Autodesk Inventor part; units mm, degrees
ref_plane "Work Plane1" through (83, 0, 0) normal (-1, 0, 0) x (0, 0, 1)
ref_plane "YZ Plane" through (0, 0, 0) normal (1, 0, 0) x (0, 1, 0)
ref_plane "XZ Plane" through (0, 0, 0) normal (0, 1, 0) x (-1, 0, 0)
sketch "Sketch1" plane through (0, 0, 0) normal (0, 0, 1) x (1, 0, 0)
  line L0 (0, 0) -> (5, 0)
  line L1 (5, 0) -> (5, -18)
  line L2 (5, -18) -> (26, -18)
  line L3 (26, -18) -> (26, 0)
  line L4 (26, 0) -> (74, 0)
  arc A0 (74, 0) -> (74, 18) centre (74, 9) ccw
  line L5 (74, 18) -> (0, 18)
  line L6 (0, 18) -> (0, 0)
  circle A1 centre (20.5, -18) radius 10.5
  dimension "d0" = 5
  dimension "d1" = 18
  dimension "d2" = 21
  dimension "d3" = 18
  dimension "d4" = 48
  dimension "d5" = 18
  dimension "d6" = 9
  dimension "d7" = 74
  dimension "d8" = 21
extrude "Extrusion1" add sketch "Sketch1" along normal blind 6
sketch "Sketch2" plane through (0, 0, 0) normal (0, 0, -1) x (-1, 0, 0)
  circle A0 centre (-74, 9) radius 4.5
  arc A1 (-26, -9.0557) -> (-10, -18) centre (-20.5, -18) ccw
  circle A2 centre (-20.5, -18) radius 4.5
  point P0 (0, 0)
  dimension "d11" = 9
  dimension "d12" = 9
extrude "Extrusion2" cut sketch "Sketch2" against normal through all
sketch "Sketch3" plane through (0, 0, 0) normal (0, 0, -1) x (-1, 0, 0)
  circle A0 centre (-7, 9) radius 1.5
  circle A1 centre (-19, 9) radius 1.5
  point P0 (0, 0)
  dimension "d16" = 3
  dimension "d17" = 3
extrude "Extrusion3" cut sketch "Sketch3" against normal through all
ref_plane "Work Plane1" through (83, 0, 0) normal (-1, 0, 0) x (0, 0, 1)
sketch "Sketch4" plane through (83, 0, 0) normal (-1, 0, 0) x (0, 0, 1)
  circle A0 centre (3, 9) radius 1.5
  point P0 (0, 0)
  dimension "d22" = 3
extrude "Extrusion4" cut sketch "Sketch4" along normal blind 18
fillet "Fillet3" radius 1 8 edges at (83, 9, 0) (50, 0, 0) (37, 18, 0) (2.5, 0, 0) (5, -9, 0) (25.6235, -27.1652, 0) (7.5, -18, 0) (26, -4.5279, 0)
sketch "Sketch5" plane through (0, 18, 6) normal (0, 1, 0) x (1, 0, 0)
  circle A0 centre (69, 2.5) radius 1.5
  circle A1 centre (58, 2.5) radius 1.5
  point P0 (0, 6)
  dimension "d26" = 3
  dimension "d27" = 3
extrude "Extrusion5" cut sketch "Sketch5" against normal blind 5
sketch "Sketch6" plane through (0, 0, 6) normal (0, 0, 1) x (1, 0, 0)
  line L0 (71, 0) -> (77, 0)
  line L1 (77, 0) -> (77, 6)
  line L2 (77, 6) -> (71, 6)
  line L3 (71, 6) -> (71, 0)
  line L4 (17.5, -18) -> (23.5, -18)
  line L5 (23.5, -18) -> (23.5, -29)
  line L6 (23.5, -29) -> (17.5, -29)
  line L7 (17.5, -29) -> (17.5, -18)
  point P0 (0, 0)
  dimension "d30" = 6
  dimension "d31" = 6
  dimension "d32" = 6
  dimension "d33" = 11
extrude "Extrusion6" cut sketch "Sketch6" against normal through all
sketch "Sketch7" plane through (0, 0, 0) normal (0, 0, -1) x (-1, 0, 0)
  arc A0 (-38.7148, 11.0023) -> (-38.2652, 13.3358) centre (-45.6076, 13.5402) ccw
  arc A1 (-38.1755, 10.6175) -> (-38.7148, 11.0023) centre (-42.3608, 5.3217) ccw
  arc A2 (-36.1152, 11.8018) -> (-38.1755, 10.6175) centre (-33.5331, 4.9255) ccw
  arc A3 (-35.5101, 11.1585) -> (-36.1152, 11.8018) centre (-42.3608, 5.3217) ccw
  arc A4 (-36.8185, 9.1746) -> (-35.5101, 11.1585) centre (-42.2153, 14.1571) ccw
  arc A5 (-36.4675, 8.6128) -> (-36.8185, 9.1746) centre (-42.3608, 5.3217) ccw
  arc A6 (-34.1108, 8.9185) -> (-36.4675, 8.6128) centre (-34.3567, 1.5774) ccw
  arc A7 (-33.798, 8.0925) -> (-34.1108, 8.9185) centre (-42.3608, 5.3217) ccw
  arc A8 (-35.7659, 6.7603) -> (-33.798, 8.0925) centre (-38.8453, 13.4288) ccw
  arc A9 (-35.6566, 6.107) -> (-35.7659, 6.7603) centre (-42.3608, 5.3217) ccw
  arc A10 (-33.3623, 5.4875) -> (-35.6566, 6.107) centre (-36.3988, -1.2006) ccw
  arc A11 (-33.3894, 4.6047) -> (-33.3623, 5.4875) centre (-42.3608, 5.3217) ccw
  arc A12 (-35.7174, 4.1271) -> (-33.3894, 4.6047) centre (-36.0104, 11.4664) ccw
  arc A13 (-35.8664, 3.4816) -> (-35.7174, 4.1271) centre (-42.3608, 5.3217) ccw
  arc A14 (-33.9838, 2.0314) -> (-35.8664, 3.4816) centre (-39.3486, -2.9857) ccw
  arc A15 (-34.3467, 1.2261) -> (-33.9838, 2.0314) centre (-42.3608, 5.3217) ccw
  arc A16 (-36.6802, 1.6757) -> (-34.3467, 1.2261) centre (-34.1423, 8.5684) ccw
  arc A17 (-37.0649, 1.1364) -> (-36.6802, 1.6757) centre (-42.3608, 5.3217) ccw
  arc A18 (-35.8806, -0.9239) -> (-37.0649, 1.1364) centre (-42.757, -3.506) ccw
  arc A19 (-36.524, -1.529) -> (-35.8806, -0.9239) centre (-42.3608, 5.3217) ccw
  arc A20 (-38.5079, -0.2207) -> (-36.524, -1.529) centre (-33.5254, 5.1762) ccw
  arc A21 (-39.0697, -0.5716) -> (-38.5079, -0.2207) centre (-42.3608, 5.3217) ccw
  arc A22 (-38.764, -2.9284) -> (-39.0697, -0.5716) centre (-46.105, -2.6824) ccw
  arc A23 (-39.59, -3.2412) -> (-38.764, -2.9284) centre (-42.3608, 5.3217) ccw
  arc A24 (-40.9222, -1.2732) -> (-39.59, -3.2412) centre (-34.2536, 1.8061) ccw
  arc A25 (-41.5755, -1.3825) -> (-40.9222, -1.2732) centre (-42.3608, 5.3217) ccw
  arc A26 (-42.1949, -3.6768) -> (-41.5755, -1.3825) centre (-48.8831, -0.6403) ccw
  arc A27 (-43.0777, -3.6497) -> (-42.1949, -3.6768) centre (-42.3608, 5.3217) ccw
  arc A28 (-43.5554, -1.3218) -> (-43.0777, -3.6497) centre (-36.2161, -1.0287) ccw
  arc A29 (-44.2008, -1.1727) -> (-43.5554, -1.3218) centre (-42.3608, 5.3217) ccw
  arc A30 (-45.6511, -3.0553) -> (-44.2008, -1.1727) centre (-50.6681, 2.3095) ccw
  arc A31 (-46.4564, -2.6925) -> (-45.6511, -3.0553) centre (-42.3608, 5.3217) ccw
  arc A32 (-46.0068, -0.3589) -> (-46.4564, -2.6925) centre (-39.114, -2.8968) ccw
  arc A33 (-46.5461, 0.0258) -> (-46.0068, -0.3589) centre (-42.3608, 5.3217) ccw
  arc A34 (-48.6064, -1.1585) -> (-46.5461, 0.0258) centre (-51.1885, 5.7179) ccw
  arc A35 (-49.2115, -0.5151) -> (-48.6064, -1.1585) centre (-42.3608, 5.3217) ccw
  arc A36 (-47.9032, 1.4688) -> (-49.2115, -0.5151) centre (-42.5063, -3.5137) ccw
  arc A37 (-48.2541, 2.0306) -> (-47.9032, 1.4688) centre (-42.3608, 5.3217) ccw
  arc A38 (-50.6108, 1.7249) -> (-48.2541, 2.0306) centre (-50.3649, 9.0659) ccw
  arc A39 (-50.9237, 2.5508) -> (-50.6108, 1.7249) centre (-42.3608, 5.3217) ccw
  arc A40 (-48.9557, 3.883) -> (-50.9237, 2.5508) centre (-45.8763, -2.7855) ccw
  arc A41 (-49.065, 4.5364) -> (-48.9557, 3.883) centre (-42.3608, 5.3217) ccw
  arc A42 (-51.3593, 5.1558) -> (-49.065, 4.5364) centre (-48.3228, 11.8439) ccw
  arc A43 (-51.3322, 6.0386) -> (-51.3593, 5.1558) centre (-42.3608, 5.3217) ccw
  arc A44 (-49.0043, 6.5163) -> (-51.3322, 6.0386) centre (-48.7112, -0.823) ccw
  arc A45 (-48.8552, 7.1617) -> (-49.0043, 6.5163) centre (-42.3608, 5.3217) ccw
  arc A46 (-50.7378, 8.612) -> (-48.8552, 7.1617) centre (-45.373, 13.629) ccw
  arc A47 (-50.3749, 9.4172) -> (-50.7378, 8.612) centre (-42.3608, 5.3217) ccw
  arc A48 (-48.0414, 8.9677) -> (-50.3749, 9.4172) centre (-50.5793, 2.0749) ccw
  arc A49 (-47.6567, 9.5069) -> (-48.0414, 8.9677) centre (-42.3608, 5.3217) ccw
  arc A50 (-48.841, 11.5673) -> (-47.6567, 9.5069) centre (-41.9646, 14.1494) ccw
  arc A51 (-48.1976, 12.1724) -> (-48.841, 11.5673) centre (-42.3608, 5.3217) ccw
  arc A52 (-46.2137, 10.864) -> (-48.1976, 12.1724) centre (-51.1962, 5.4671) ccw
  arc A53 (-45.6519, 11.215) -> (-46.2137, 10.864) centre (-42.3608, 5.3217) ccw
  arc A54 (-45.9576, 13.5717) -> (-45.6519, 11.215) centre (-38.6166, 13.3258) ccw
  arc A55 (-45.1317, 13.8845) -> (-45.9576, 13.5717) centre (-42.3608, 5.3217) ccw
  arc A56 (-43.7995, 11.9166) -> (-45.1317, 13.8845) centre (-50.468, 8.8372) ccw
  arc A57 (-43.1461, 12.0258) -> (-43.7995, 11.9166) centre (-42.3608, 5.3217) ccw
  arc A58 (-42.5267, 14.3201) -> (-43.1461, 12.0258) centre (-35.8385, 11.2837) ccw
  arc A59 (-41.6439, 14.2931) -> (-42.5267, 14.3201) centre (-42.3608, 5.3217) ccw
  arc A60 (-41.1662, 11.9651) -> (-41.6439, 14.2931) centre (-48.5055, 11.6721) ccw
  arc A61 (-40.5208, 11.816) -> (-41.1662, 11.9651) centre (-42.3608, 5.3217) ccw
  arc A62 (-39.0705, 13.6987) -> (-40.5208, 11.816) centre (-34.0535, 8.3339) ccw
  arc A63 (-38.2652, 13.3358) -> (-39.0705, 13.6987) centre (-42.3608, 5.3217) ccw
  circle A64 centre (-42.3608, 5.3217) radius 1.5
  point P0 (0, 0)
  dimension "d36" = 3
extrude "Extrusion7" cut sketch "Sketch7" against normal through all contours A64
properties part number "Hand - Digit 0-1" material "ABS Plastic"
The model under review builds one solid part; all positions refer to its coordinate system, in mm. A direction names the side the tool comes from. Give positions to 0.01 mm unless a question says otherwise; leave off trailing zeros. Loops run counter-clockwise (first coordinate to the right, second up) from the corner with the lowest first, then second, coordinate; pieces in that order, holes last. Notation, with made-up numbers: (-1, 76) -> (47, 76) arc R25 cw to (47, 91) -> close; hole circle Ø5 at (61.25, -1.75). An arc over 180 degrees is marked (long way). Answer as a JSON object with one key per item and string values. Group by question number.
Q1. Take a section at B-B (x = 58). Write out the cut boundary in (y, z).
Q2. Draft analysis for pull direction X (two halves, no side actions). For faces 5 (the flat face through (65, 9, 3)), 6 (the cylindrical face through (8.2, 8.1, 3)), 7 (the cylindrical face through (80.655, 10.464, 2.675)), 8 (the flat face through (5, -9, 3)), state which applies: pulls with the +X half, pulls with the -X half, needs draft (parallel to the pull), parting line crosses it, or undercut.
Q3. Take a section at A-A (x = 7). Write out the cut boundary in (y, z).
Q4. Insertion check: pin 1 (1 mm diameter, centred on y = -11.5, z = 0.5, fed in from +X); pin 2 (1 mm diameter, centred on y = -11, z = 1.5, fed in from +X); pin 3 (2.5 mm diameter, centred on y = -12.5, z = 2.5, fed in from -X); pin 4 (5.5 mm diameter, centred on x = 20.5, y = -18, fed in from -Z). Each pin has a flat end and moves straight along its axis. Give the tip position at first contact, or say it passes through.
Q5. Tool access review of faces 1 (the cylindrical face through (59.43, 15.54, 3.05)), 2 (the cylindrical face through (67.412, 10.464, 2.675)), 3 (the flat face through (71, 3, 3)), 4 (the cylindrical face through (12.14, -24.35, 3.46)): name each direction out of +Z, -Z, +X, -X, +Y, -Y from which nothing blocks a thin tool from reaching the whole face with its end or side.
Q6. Wall thickness on line 1 along Y through (x, z) = (7, 3); line 2 along Z through (x, y) = (66, 9); line 3 along X through (y, z) = (-3.5, 3): over which ranges is each line inside the solid? List them lowest first.
Answer below:
{
 "1": {"outline": "(0, 1) arc R1 ccw to (1, 0) -> (17, 0) arc R1 ccw to (18, 1) -> (18, 2) -> (13, 2) -> (13, 5) -> (18, 5) -> (18, 6) -> (0, 6) -> close"},
 "2": {"face 5": "pulls with the +X half", "face 6": "undercut", "face 7": "needs draft", "face 8": "pulls with the -X half"},
 "3": {"outline": "(-18, 1) arc R1 ccw to (-17, 0) -> (7.5, 0) -> (7.5, 6) -> (-18, 6) -> close; (10.5, 0) -> (17, 0) arc R1 ccw to (18, 1) -> (18, 6) -> (10.5, 6) -> close"},
 "4": {"pin 1": "stops at x = 29.03", "pin 2": "stops at x = 28.75", "pin 3": "stops at x = 5", "pin 4": "passes through"},
 "5": {"face 1": "+Y", "face 2": "+X", "face 3": "+Z, -Z, -Y", "face 4": "+Z, -Z, -X, -Y"},
 "6": {"line 1": "y = -18 to 7.5, 10.5 to 18", "line 2": "z = 0 to 1.5, 4.5 to 6", "line 3": "x = 5 to 26"}
}
